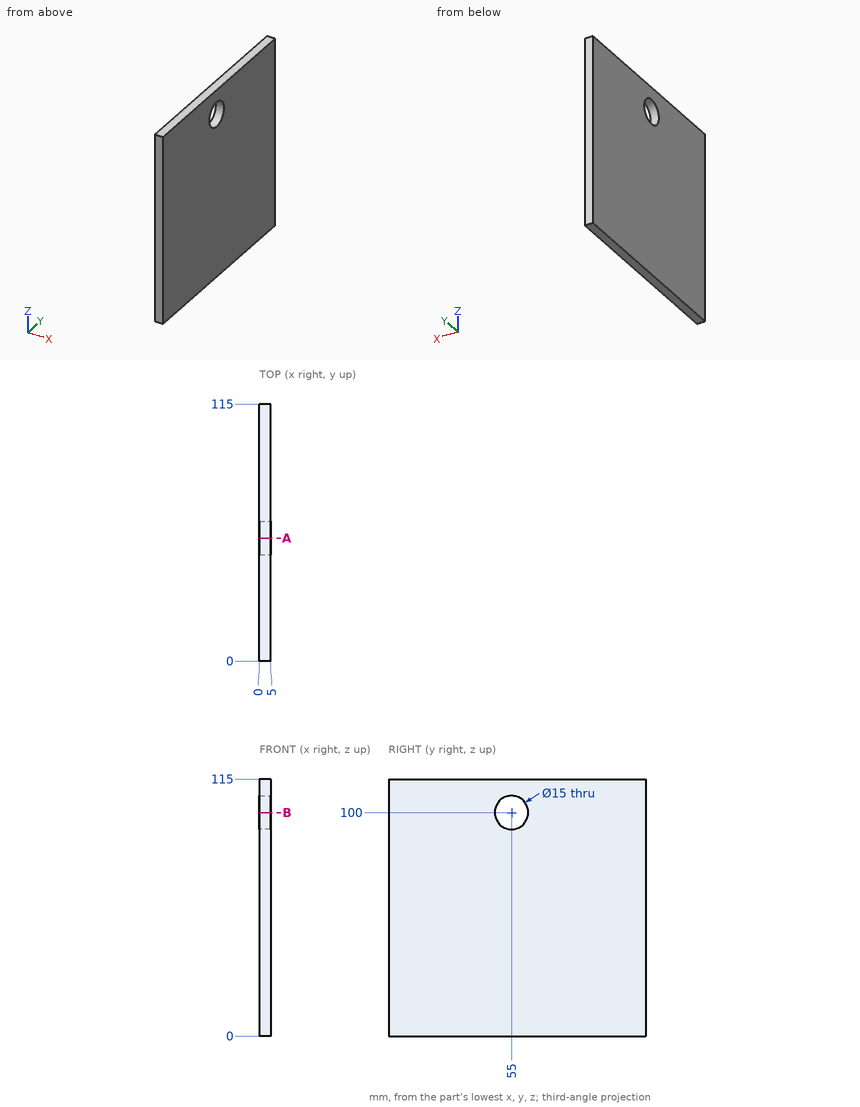
Design review of the part shown in the three views and the two pictorial views. Dimensions are in mm from the part's minimum x, y and z. Coordinates: 2 decimals unless noted, no trailing zeros. Write each loop counter-clockwise with the first axis right and the second up, starting at its lowest first coordinate (ties: lowest second). Pieces come first, ordered by that corner, then holes. Notation, with made-up numbers: (78.25, 17.5) - (123.25, 17.5) arc R14 ccw to (123.25, 32.5) - close; hole circle Ø6 at (5, -15). An arc over 180 degrees is marked (long way). Write item = value, one per line.
(1) Consider section A-A, the plane y = 55. Give the boundary of the cut face in (x, z).
Result sheet:
outline = (0, 0) - (5, 0) - (5, 92.5) - (0, 92.5) - close; (0, 107.5) - (5, 107.5) - (5, 115) - (0, 115) - close
(2) Consider section B-B, the plane z = 100. Give the boundary of the cut face in (x, y), then the cut area to 3 significant figures.
Result sheet:
outline = (0, 0) - (5, 0) - (5, 47.5) - (0, 47.5) - close; (0, 62.5) - (5, 62.5) - (5, 115) - (0, 115) - close
area = 500 mm^2
(3) For line 1 (Y direction, x = 1.55, z = 100); line 2 (Z direction, x = 0.95, y = 54.5); line 3 (Z direction, x = 1.15, y = 58), list the stretches that pass through material, from the lowest coordinate up. Write a range as [from, to].
Result sheet:
line_1 = [0, 47.5], [62.5, 115]
line_2 = [0, 92.52], [107.48, 115]
line_3 = [0, 93.13], [106.87, 115]
